```python
from build123d import *

# Parameters (mm, degrees)
F0_W     = 12.7
F0_H     = 38.1
F1_DEPTH = 25.4
F2_R     = 5.08
F3_R     = 2.54
F4_R     = 5.08


with BuildPart() as f1:
    # F0 (on Top) → F1 (new body)
    with BuildSketch(Plane.XY):
        with BuildLine():
            Line((5.467289, 31.414881), (-7.232711, 31.414881))
            Line((-7.232711, 31.414881), (-7.232711, -95.585119))
            ThreePointArc((-7.232711, -95.585119), (-42.453229, -130.805637), (-77.673748, -95.585119))
            Line((-77.673748, -95.585119), (-90.373748, -95.585119))
            ThreePointArc((-90.373748, -95.585119), (-42.453229, -143.505637), (5.467289, -95.585119))
            Line((5.467289, -95.585119), (5.467289, 31.414881))
        make_face()
        Polygon((-7.232711, 44.114881), (-7.232711, 31.414881), (5.467289, 31.414881), (24.517289, 31.414881), (37.217289, 31.414881), (37.217289, 44.114881), align=None)
        with Locations((30.867289, 12.364881)):
            Rectangle(F0_W, F0_H)
    extrude(amount=F1_DEPTH)

    # F2
    f2_edges = [f1.edges().sort_by_distance(p)[0] for p in [
        (37.217289, -6.685119, 12.7),
        (24.517289, -6.685119, 12.7),
        (37.217289, 44.114881, 12.7),
        (-7.232711, 44.114881, 12.7),
    ]]
    fillet(f2_edges, radius=F2_R)

    # F3
    f3_edges = [f1.edges().sort_by_distance(p)[0] for p in [
        (5.467289, 31.414881, 12.7),
        (24.517289, 31.414881, 12.7),
    ]]
    fillet(f3_edges, radius=F3_R)

    # F4
    f4_edges = [f1.edges().sort_by_distance(p)[0] for p in [
        (24.517289, 13.634881, 25.4),
        (23.77334, 30.670933, 25.4),
        (26.005187, -5.197221, 25.4),
        (14.992289, 31.414881, 25.4),
        (30.867289, -6.685119, 25.4),
        (6.211238, 30.670933, 25.4),
        (35.729392, -5.197221, 25.4),
        (5.467289, -33.355119, 25.4),
        (37.217289, 18.714881, 25.4),
        (-42.453229, -143.505637, 25.4),
        (35.729392, 42.626984, 25.4),
        (-84.023748, -95.585119, 25.4),
        (14.992289, 44.114881, 25.4),
        (-42.453229, -130.805637, 25.4),
        (-5.744813, 42.626984, 25.4),
        (-7.232711, -28.275119, 25.4),
        (24.517289, 13.634881, 0),
        (23.77334, 30.670933, 0),
        (26.005187, -5.197221, 0),
        (14.992289, 31.414881, 0),
        (30.867289, -6.685119, 0),
        (6.211238, 30.670933, 0),
        (35.729392, -5.197221, 0),
        (5.467289, -33.355119, 0),
        (37.217289, 18.714881, 0),
        (-42.453229, -143.505637, 0),
        (35.729392, 42.626984, 0),
        (-84.023748, -95.585119, 0),
        (14.992289, 44.114881, 0),
        (-42.453229, -130.805637, 0),
        (-5.744813, 42.626984, 0),
        (-7.232711, -28.275119, 0),
    ]]
    fillet(f4_edges, radius=F4_R)


solid = f1.part
```
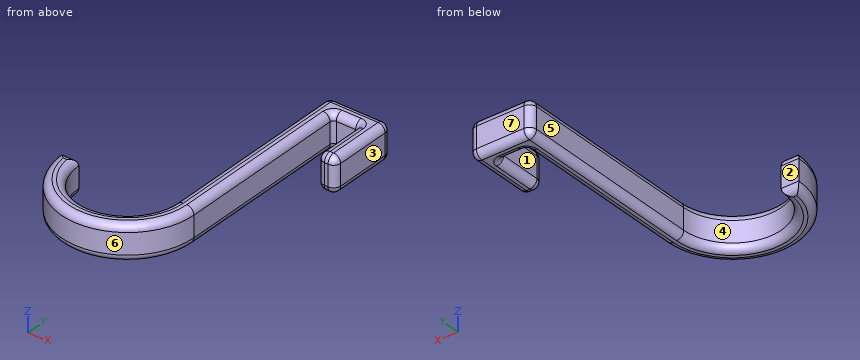
The listing builds one solid part. Answer for the finished solid, in the listing's coordinates (mm). Face numbers are marked on the shaded views. A direction names the side the tool comes from. Give positions to 0.01 mm unless a question says otherwise; leave off trailing zeros. Loops run counter-clockwise (first coordinate to the right, second up) from the corner with the lowest first, then second, coordinate; pieces in that order, holes last. Notation, with made-up numbers: M 66,46 L 114,46 A18 cw 114,79 Z; hole C 68,52.25 d9. An arc over 180 degrees is marked long. One line per item, written item: value.
Q1. A cutting plane is placed at B-B on z = 15.5. Determine the outline of the cut face in (x, y).
Working result:
outline: M -90.37,-95.59 A47.92 ccw 5.47,-95.59 L 5.47,28.87 A2.54 cw 8.01,31.41 L 21.98,31.41 A2.54 cw 24.52,28.87 L 24.52,-1.61 A5.08 ccw 29.6,-6.69 L 32.14,-6.69 A5.08 ccw 37.22,-1.61 L 37.22,39.03 A5.08 ccw 32.14,44.11 L -2.15,44.11 A5.08 ccw -7.23,39.03 L -7.23,-95.59 A35.22 cw -77.67,-95.59 Z
Q2. A cutting plane is placed at C-C on z = 3.25. Determine the outline of the cut face in (x, y), then the cut area to 3 significant figures.
Working result:
outline: M -90.03,-95.93 A47.58 ccw 5.13,-95.59 L 5.13,28.87 A2.88 cw 8.01,31.76 L 21.98,31.76 A2.88 cw 24.86,28.87 L 24.86,-1.61 A4.74 ccw 29.6,-6.34 L 32.14,-6.34 A4.74 ccw 36.88,-1.61 L 36.88,39.03 A4.74 ccw 32.14,43.77 L -2.15,43.77 A4.74 ccw -6.89,39.03 L -6.89,-95.59 A35.56 cw -78.01,-95.93 Z
area: 4,060 mm^2
Q3. For the marked faces 1, 2 and 3, determine the directions among +Z, -Z, +X, -X, +Y, -Y from which every point of the face is accessible in a straight line to the end or side of a thin tool.
Working result:
face 1: +Z, -Z, -Y
face 2: +Z, -Z, -X, +Y
face 3: +Z, -Z, +X, +Y, -Y
Q4. Find the intervals of material crossed by line 1 (X direction, y = 14, z = 8.5); line 2 (X direction, y = -18, z = 6.5); line 3 (X direction, y = -104.5, z = 1.5), in increasing order. Write a range as from..to.
Working result:
line 1: x = -7.23..5.47, 24.52..37.22
line 2: x = -7.23..5.47
line 3: x = -88.03..-78.05, -6.86..3.13
Q5. A cutting plane is placed at A-A on y = -70.5. Determine the outline of the cut face in (x, z), then the cut area to 3 significant figures.
Working result:
outline: M -7.23,5.08 A5.08 ccw -2.15,0 L 0.39,0 A5.08 ccw 5.47,5.08 L 5.47,20.32 A5.08 ccw 0.39,25.4 L -2.15,25.4 A5.08 ccw -7.23,20.32 Z
area: 300 mm^2
Q6. Determine the mould class of the marked faces 4, 5, 6 and 7 for opening direction X: +X half, -X half, draft (parallel to the pull), parting line (faces both ways), or undercut.
Working result:
face 4: undercut
face 5: -X half
face 6: parting line
face 7: draft
Q7. Flat-ended cylindrical pins translate along their axes: P1, Ø4.5, axis at y = 0, z = 15.5, coming from the -X side; P2, Ø12, axis at x = -19.5, z = 13.5, coming from the -Y side; P3, Ø3, axis at x = 17.5, z = 22, coming from the +Y side. Find the tip coordinate at first contact, or state that the pin passes through.
Working result:
P1: stops at x = -7.23
P2: stops at y = -140.41
P3: stops at y = 44.11
